The drawing under review shows one solid part. Ordinate dimensions are in mm from its lowest x, y, z. A direction names the side the tool comes from. Give positions to 0.01 mm unless a question says otherwise; leave off trailing zeros. Write each loop counter-clockwise with the first axis right and the second up, starting at its lowest first coordinate (ties: lowest second). Pieces come first, ordered by that corner, then holes.
Q1. We need section A-A (y = 2). Write out the cut boundary in (x, z).
Q2. Insertion check: P1, Ø2.5, axis at x = 7, y = 6.5, coming from the +Z side; P2, Ø0.6, axis at x = 1, z = 7.5, coming from the +Y side; P3, Ø1, axis at x = 11, y = 12, coming from the +Z side. Each pin has a flat end and moves straight along its axis. Give the tip position at first contact, or say it passes through.
Q3. Mouldability with a two-part tool opening along Z and no side actions: class the marked faces 4, 5 and 6 as released by +Z, released by -Z, zero draft, split by the parting line, or undercut.
Q4. We need section D-D (y = 11.5). Write out the cut boundary in (x, z).
Q5. Machinability: for the marked faces 1, 2 and 3, which of the approach directions +Z, -Z, +X, -X, +Y, -Y give a long, thin tool a straight path to every point of the face, cutting with its end or side? Answer none if there is none.
Q6. We need section B-B (z = 6). Write out the cut boundary in (x, y), then the cut area to 3 significant figures.
Q7. We need section C-C (x = 1.5). Write out the cut boundary in (y, z), then the cut area to 3 significant figures.
Q8. For line 1 (Z direction, x = 11.2, y = 2); line 2 (X direction, y = 1.5, z = 10); line 3 (Z direction, x = 9, y = 10.5), list the stretches that pass through material, from the lowest coordinate up.
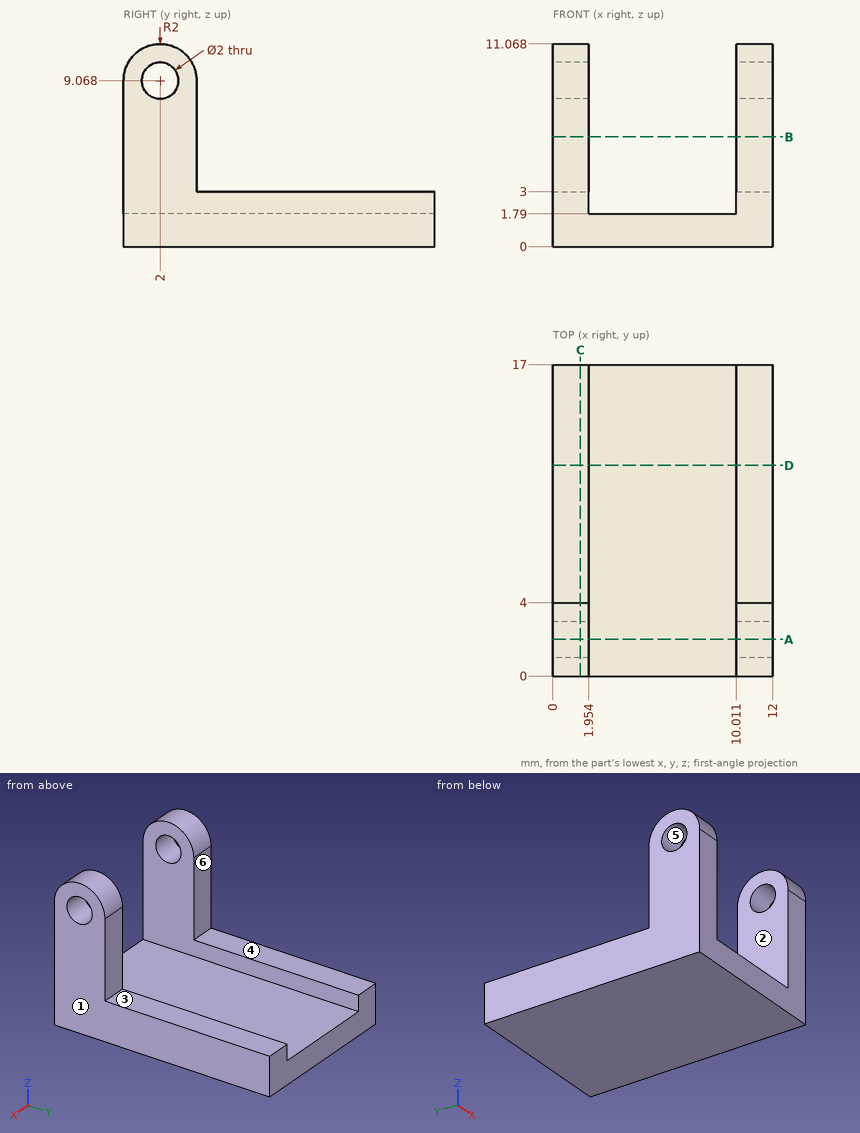
Computed:
1. outline: (0, 0) - (12, 0) - (12, 8.07) - (10.01, 8.07) - (10.01, 1.79) - (1.95, 1.79) - (1.95, 8.07) - (0, 8.07) - close; (0, 10.07) - (1.95, 10.07) - (1.95, 11.07) - (0, 11.07) - close; (10.01, 10.07) - (12, 10.07) - (12, 11.07) - (10.01, 11.07) - close
2. P1: stops at z = 1.79
2. P2: stops at y = 4
2. P3: stops at z = 3
3. face 4: released by +Z
3. face 5: undercut
3. face 6: zero draft
4. outline: (0, 0) - (12, 0) - (12, 3) - (10.01, 3) - (10.01, 1.79) - (1.95, 1.79) - (1.95, 3) - (0, 3) - close
5. face 1: +Z, -Z, +X, +Y, -Y
5. face 2: +Z, +Y, -Y
5. face 3: +Z, +X, -X, +Y
6. outline: (0, 0) - (1.95, 0) - (1.95, 4) - (0, 4) - close; (10.01, 0) - (12, 0) - (12, 4) - (10.01, 4) - close
6. area: 15.8 mm2
7. outline: (0, 0) - (17, 0) - (17, 3) - (4, 3) - (4, 9.07) arc R2 ccw to (0, 9.07) - close; hole circle Ø2 at (2, 9.07)
7. area: 78.4 mm2
8. line 1: z = 0 to 8.07, 10.07 to 11.07
8. line 2: x = 0 to 1.95, 10.01 to 12
8. line 3: z = 0 to 1.79
